from build123d import *

# Parameters (mm, degrees)
F2_DEPTH  = 72
F3_W      = 72
F3_H      = 22
F4_DEPTH  = 6
F6_DEPTH  = 25.001
F8_DEPTH  = 12
F10_DEPTH = 12
F11_R     = 12
F12_DEPTH = 134.001


with BuildPart() as f2:
    # F0 (on Front) → F2 (new body)
    with BuildSketch(Plane.XZ):
        Polygon((-134, 11), (-146, 11), (-146, -19), (-74, -19), (-74, -25), (0, -25), (0, 0), (-115, 0), (-115, 65), (-146, 65), (-146, 41), (-134, 41), align=None)
    extrude(amount=-F2_DEPTH)

    # F3 (on face) → F4 (join)
    with BuildSketch(Plane(origin=(0, 0, -19), x_dir=(1, 0, 0), z_dir=(0, 0, -1))):
        with Locations((-110, -61)):
            Rectangle(F3_W, F3_H)
    extrude(amount=F4_DEPTH)

    # F5 (on Top) → F6 (cut, through all)
    with BuildSketch(Plane.XY):
        with BuildLine():
            Line((-50, 24), (0, 24))
            Line((0, 24), (0, 48))
            Line((0, 48), (-50, 48))
            ThreePointArc((-50, 48), (-62, 36), (-50, 24))
        make_face()
    extrude(amount=-F6_DEPTH, mode=Mode.SUBTRACT)

    # F7 (on face) → F8 (cut)
    with BuildSketch(Plane(origin=(-146, 0, 0), x_dir=(0, -1, 0), z_dir=(-1, 0, 0))):
        with BuildLine():
            Line((-13.861853, 11), (-58.138147, 11))
            ThreePointArc((-58.138147, 11), (-36, 1.246048), (-13.861853, 11))
        make_face()
    extrude(amount=-F8_DEPTH, mode=Mode.SUBTRACT)

    # F9 (on face) → F10 (cut)
    with BuildSketch(Plane(origin=(-146, 0, 0), x_dir=(0, -1, 0), z_dir=(-1, 0, 0))):
        with BuildLine():
            Line((-60, 41), (-12, 41))
            ThreePointArc((-12, 41), (-36, 53), (-60, 41))
        make_face()
        with BuildLine():
            Line((-6.492059, 17.588768), (-8.615558, 35.251218))
            ThreePointArc((-8.615558, 35.251218), (-10.147489, 38.219976), (-12, 41))
            Line((-12, 41), (-60, 41))
            ThreePointArc((-60, 41), (-48.025215, -4.484436), (-6.492059, 17.588768))
        make_face()
    extrude(amount=-F10_DEPTH, mode=Mode.SUBTRACT)

    # F11 (on face) → F12 (cut, through all)
    with BuildSketch(Plane(origin=(-134, 0, 0), x_dir=(0, -1, 0), z_dir=(-1, 0, 0))):
        with Locations((-36, 23)):
            Circle(F11_R)
    extrude(amount=-F12_DEPTH, mode=Mode.SUBTRACT)


solid = f2.part
Geometry check sheet. Reference: the model listing, model coordinates, mm. A direction names the side the tool comes from. Round coordinates to 2 decimals unless told otherwise and drop trailing zeros. Write each loop counter-clockwise with the first axis right and the second up, starting at its lowest first coordinate (ties: lowest second). Pieces come first, ordered by that corner, then holes.
Item 1: Section check A-A (z = 23). Record the boundary of the cut face in (x, y), plus the area to 3 significant figures.
Determined:
outline: (-134, 0) - (-115, 0) - (-115, 24) - (-134, 24) - close; (-134, 48) - (-115, 48) - (-115, 72) - (-134, 72) - close
area: 912 mm2
Item 2: Go/stop test with flat-tipped pins: pin 1 Ø10 at (y, z) = (33.5, 52) entering from +X; pin 2 Ø1 at (y, z) = (13, 24) entering from -X; pin 3 Ø6 at (x, y) = (-138, 5) entering from -Z. Record where each tip stops, or that it passes through.
Determined:
pin 1: stops at x = -115
pin 2: stops at x = -134
pin 3: stops at z = -19
Item 3: Section check D-D (z = -17). Record the boundary of the cut face in (x, y).
Determined:
outline: (-146, 0) - (0, 0) - (0, 24) - (-50, 24) arc R12 cw to (-50, 48) - (0, 48) - (0, 72) - (-146, 72) - close
Item 4: Material ranges on line 1 along Z through (x, y) = (-119.5, 36); line 2 along Z through (x, y) = (-52.5, 56); line 3 along X through (y, z) = (12.5, 8), recorded low to high.
Determined:
line 1: z = -19 to 11, 35 to 65
line 2: z = -25 to 0
line 3: x = -134 to -115
Item 5: Mould release check, pull along Z, two halves, no side actions. Record for faces 1 (the face through (-146, 37, -11)), 2 (the face through (-140, 66, 41)), 3 (the face through (-58, 51, -25)): +Z half, -Z half, draft (parallel to the pull), parting line (faces both ways), or undercut.
Determined:
face 1: draft
face 2: undercut
face 3: -Z half
Item 6: Section check B-B (x = -17.5). Record the boundary of the cut face in (y, z).
Determined:
outline: (0, -25) - (24, -25) - (24, 0) - (0, 0) - close; (48, -25) - (72, -25) - (72, 0) - (48, 0) - close
Item 7: Section check C-C (y = 36). Record the boundary of the cut face in (x, z).
Determined:
outline: (-146, -19) - (-74, -19) - (-74, -25) - (-62, -25) - (-62, 0) - (-115, 0) - (-115, 11) - (-134, 11) - (-134, -7) - (-146, -7) - close; (-146, 53) - (-134, 53) - (-134, 35) - (-115, 35) - (-115, 65) - (-146, 65) - close
Item 8: Access from +Z, -Z, +X, -X, +Y, -Y to the whole of each face (thin tool, end or side, straight path). Record for faces 4 (the face through (-115, 35, 39)), 5 (the face through (-140, 36, -7)), 6 (the face through (-111, 50, -22)), 7 (the face through (-25, 48, -12)), 8 (the face through (-140, 68, 11)).
Determined:
face 4: +Z, +X, +Y, -Y
face 5: -X
face 6: -Z, -X, -Y
face 7: +Z, -Z, +X
face 8: -X, +Y, -Y
